```python
from build123d import *

# Parameters (mm, degrees)
SKETCH1_R                    = 5.5
BOSS_EXTRUDE1_DEPTH          = 38
SKETCH8_R                    = 7.5
BOSS_EXTRUDE2_DEPTH          = 1.5
SKETCH9_R                    = 6
BOSS_EXTRUDE3_DEPTH          = 5
SKETCH2_R                    = 4
CUT_EXTRUDE1_DEPTH           = 18
KEYWAY_SLOT_DEPTH            = 2.5
SKETCH11_OUTSIDE_W           = 25.704
SKETCH11_OUTSIDE_H           = 25.704
SKETCH11_OUTSIDE_R           = 5
TRIM_FOR_M10_WHEEL_NUT_DEPTH = 10


with BuildPart() as part:
    # Sketch1 → Boss-Extrude1 (new body)
    with BuildSketch(Plane.XY):
        Circle(SKETCH1_R)
    extrude(amount=BOSS_EXTRUDE1_DEPTH)

    # Sketch8 → Boss-Extrude2 (add)
    with BuildSketch(Plane.XY.offset(38)):
        Circle(SKETCH8_R)
    extrude(amount=-BOSS_EXTRUDE2_DEPTH)

    # Sketch9 → Boss-Extrude3 (add)
    with BuildSketch(Plane(origin=(0, 0, 36.5), x_dir=(-1, 0, 0), z_dir=(0, 0, -1))):
        with Locations(Location((0, 0, 0), (0, 0, 180))):
            Circle(SKETCH9_R)
    extrude(amount=BOSS_EXTRUDE3_DEPTH)

    # Sketch2 → Cut-Extrude1 (cut)
    with BuildSketch(Plane.XY.offset(38)):
        Circle(SKETCH2_R)
    extrude(amount=-CUT_EXTRUDE1_DEPTH, mode=Mode.SUBTRACT)

    # Sketch7 → Keyway slot (cut)
    with BuildSketch(Plane(origin=(0, 5.5, 0), x_dir=(1, 0, 0), z_dir=(0, 1, 0))):
        with BuildLine():
            Line((-2, -29), (-2, -23))
            ThreePointArc((-2, -23), (0, -21), (2, -23))
            Line((2, -23), (2, -29))
            ThreePointArc((2, -29), (0, -31), (-2, -29))
        make_face()
    extrude(amount=-KEYWAY_SLOT_DEPTH, mode=Mode.SUBTRACT)

    # Sketch11 outside → Trim for M10 wheel nut (cut)
    with BuildSketch(Plane(origin=(0, 0, 0), x_dir=(-1, 0, 0), z_dir=(0, 0, -1))):
        Rectangle(SKETCH11_OUTSIDE_W, SKETCH11_OUTSIDE_H)
        Circle(SKETCH11_OUTSIDE_R, mode=Mode.SUBTRACT)
    extrude(amount=-TRIM_FOR_M10_WHEEL_NUT_DEPTH, mode=Mode.SUBTRACT)


solid = part.part
```
Here's how the part is built. I have some questions about the finished solid (model axes, mm). A direction names the side the tool comes from. Round coordinates to 2 decimals unless told otherwise and drop trailing zeros. Order: outer loops, then holes, each group sorted by start corner. A loop starts at its lowest first (then second) coordinate and runs counter-clockwise, first axis right, second up. Notation, with made-up numbers: (-27, 85) -> (-23, 85) arc R19 cw to (-23, 118) -> close; hole circle Ø2 at (29, -8). An arc over 180 degrees is marked (long way). Use a Markdown table: item, result. Add a question column.
(1) Suppose I cut it at D-D, the plane y = 0. Please give me the cut outline in (x, z).
(2) For pin 1 Ø4 at (x, y) = (0.5, 0.5) entering from +Z; pin 2 Ø1.3 at (y, z) = (4.5, 26) entering from +X; pin 3 Ø1 at (y, z) = (0, 32.5) entering from +X, each with a flat end and sliding along its axis, tell me the tip position at first contact or that it passes through.
(3) Suppose I cut it at C-C, the plane z = 23.5. Please give me the cut outline in (x, y), and give its area (3 significant figures).
(4) Suppose I cut it at B-B, the plane y = 4.5. Please give me the cut outline in (x, z).
(5) For faces 1 (the face through (0, 0, 20)), 2 (the face through (0, 4.5, 31)), 3 (the face through (1.08, -4.88, 4.93)), which set-ups out of +Z, -Z, +X, -X, +Y, -Y let a thin tool reach every point of the face, with its end or its side?
(6) I need wall thicknesses on line 1 along Y through (x, z) = (0, 33.25); line 2 along Z through (x, y) = (-6.5, -2.75); line 3 along Z through (x, y) = (1.25, 3.5). Which ranges of each line are inside material? Lowest first, please.
(7) If we mould it in two halves opening along X, with no side actions, what happens to faces 4 (the face through (0, 0, 0)), 5 (the face through (2, 4, 26)), 6 (the face through (5.723, -1.802, 34.035))? For each: released by +X, released by -X, zero draft, split by the parting line, or undercut.
(8) Suppose I cut it at A-A, the plane x = 0. Please give me the cut outline in (y, z), and give its area (3 significant figures).
Verdict:
| question | item | result |
|---|---|---|
| 1 | outline | (-7.5, 36.5) -> (-6, 36.5) -> (-6, 31.5) -> (-5.5, 31.5) -> (-5.5, 10) -> (-5, 10) -> (-5, 0) -> (5, 0) -> (5, 10) -> (5.5, 10) -> (5.5, 31.5) -> (6, 31.5) -> (6, 36.5) -> (7.5, 36.5) -> (7.5, 38) -> (4, 38) -> (4, 20) -> (-4, 20) -> (-4, 38) -> (-7.5, 38) -> close |
| 2 | pin 1 | z = 20 |
| 2 | pin 2 | x = 3.93 |
| 2 | pin 3 | x = 6 |
| 3 | outline | (-2, 3.46) -> (-2, 5.12) arc R5.5 ccw (long way) to (2, 5.12) -> (2, 3.46) arc R4 cw (long way) to start |
| 3 | area | 38.6 mm2 |
| 4 | outline | (-6, 36.5) -> (-3.97, 36.5) -> (-3.97, 31.5) -> (-3.16, 31.5) -> (-3.16, 10) -> (-2.18, 10) -> (-2.18, 0) -> (2.18, 0) -> (2.18, 10) -> (3.16, 10) -> (3.16, 31.5) -> (3.97, 31.5) -> (3.97, 36.5) -> (6, 36.5) -> (6, 38) -> (-6, 38) -> close; hole (-2, 23) arc R2 ccw to (2, 23) -> (2, 29) arc R2 ccw to (-2, 29) -> close |
| 5 | face 1 | +Z |
| 5 | face 2 | +Y |
| 5 | face 3 | -Z |
| 6 | line 1 | -6 to -4, 4 to 6 |
| 6 | line 2 | 36.5 to 38 |
| 6 | line 3 | 0 to 20 |
| 7 | face 4 | zero draft |
| 7 | face 5 | undercut |
| 7 | face 6 | split by the parting line |
| 8 | outline | (-7.5, 36.5) -> (-6, 36.5) -> (-6, 31.5) -> (-5.5, 31.5) -> (-5.5, 10) -> (-5, 10) -> (-5, 0) -> (5, 0) -> (5, 10) -> (5.5, 10) -> (5.5, 21) -> (4, 21) -> (4, 20) -> (-4, 20) -> (-4, 38) -> (-7.5, 38) -> close; (4, 31) -> (5.5, 31) -> (5.5, 31.5) -> (6, 31.5) -> (6, 36.5) -> (7.5, 36.5) -> (7.5, 38) -> (4, 38) -> close |
| 8 | area | 260 mm2 |
